The listing builds one solid part. Answer for the finished solid, in the listing's coordinates (mm). Give positions to 0.01 mm unless a question says otherwise; leave off trailing zeros. Order: outer loops, then holes, each group sorted by start corner. A loop starts at its lowest first (then second) coordinate and runs counter-clockwise, first axis right, second up.
```python
from build123d import *

# Parameters (mm, degrees)
SKETCH1_W           = 58
SKETCH1_H           = 61
SKETCH1_R           = 18
BOSS_EXTRUDE1_DEPTH = 8
SKETCH26_R          = 12.25
SKETCH26_R_2        = 3.500000003
SKETCH26_R_3        = 2.7
CUT_EXTRUDE25_DEPTH = 80


with BuildPart() as part:
    # Sketch1 → Boss-Extrude1 (new body)
    with BuildSketch(Plane.XY):
        with Locations((-375.83204095, -9.5)):
            Rectangle(SKETCH1_W, SKETCH1_H)
        with Locations((-375.83204095, -9.5)):
            Circle(SKETCH1_R, mode=Mode.SUBTRACT)
    extrude(amount=BOSS_EXTRUDE1_DEPTH)

    # Sketch26 → Cut-Extrude25 (cut)
    with BuildSketch(Plane(origin=(-392.722155748, 41.581437247, 68), x_dir=(-1, 0, 0), z_dir=(0, 0, 1))):
        with Locations((-16.890114798, 51.081437247)):
            Circle(SKETCH26_R)
        with Locations(Location((-38.640114797, 75.581437247, 0), (0, 0, 180))):
            Circle(SKETCH26_R_2)
        with Locations(Location((4.859885202, 75.581437247, 0), (0, 0, 180))):
            Circle(SKETCH26_R_2)
        with Locations(Location((-38.640114797, 26.581437247, 0), (0, 0, 180))):
            Circle(SKETCH26_R_2)
        with Locations(Location((4.859885202, 26.581437247, 0), (0, 0, 180))):
            Circle(SKETCH26_R_2)
        with Locations((-16.890114798, 16.121848563)):
            Circle(SKETCH26_R_3)
    extrude(amount=-CUT_EXTRUDE25_DEPTH, mode=Mode.SUBTRACT)


solid = part.part
```
1) Find section A-A (y = -9.5). Write down the section's boundary in (x, z).
Geometry says:
outline: (-404.83, 0) - (-393.83, 0) - (-393.83, 8) - (-404.83, 8) - close; (-357.83, 0) - (-346.83, 0) - (-346.83, 8) - (-357.83, 8) - close
2) Find section B-B (y = 15). Write down the section's boundary in (x, z).
Geometry says:
outline: (-404.83, 0) - (-401.08, 0) - (-401.08, 8) - (-404.83, 8) - close; (-394.08, 0) - (-357.58, 0) - (-357.58, 8) - (-394.08, 8) - close; (-350.58, 0) - (-346.83, 0) - (-346.83, 8) - (-350.58, 8) - close
3) Straight lines are drawn through the part: probe 1 along X at (y, z) = (12, 1); probe 2 along Y at (x, z) = (-394.5, 3.5); probe 3 along X at (y, z) = (14.5, 2). For each, find the intervals that lie inside material, in ascending order.
Geometry says:
probe 1: x = -404.83 to -399.38, -395.78 to -355.88, -352.28 to -346.83
probe 2: y = -40 to -35.66, -32.34 to 13.34, 16.66 to 21
probe 3: x = -404.83 to -401.05, -394.12 to -357.55, -350.62 to -346.83
4) Find section D-D (z = 1.75). Write down the section's boundary in (x, y).
Geometry says:
outline: (-404.83, -40) - (-346.83, -40) - (-346.83, 21) - (-404.83, 21) - close; hole circle Ø7 at (-397.58, -34); hole circle Ø7 at (-397.58, 15); hole circle Ø36 at (-375.83, -9.5); hole circle Ø7 at (-354.08, -34); hole circle Ø7 at (-354.08, 15)
5) For a pull along Y with two mould halves and no side action, classify faces 1 (the flat face through (-363, 4, 8)), 2 (the flat face through (-376, 21, 4)), 3 (the cylindrical face through (-393.815, -8.709, 3.944)) as +Y half, -Y half, draft (parallel to the pull), parting line (faces both ways), or undercut.
Geometry says:
face 1: draft
face 2: +Y half
face 3: undercut
6) Find section C-C (x = -370). Write down the section's boundary in (y, z).
Geometry says:
outline: (-40, 0) - (-26.53, 0) - (-26.53, 8) - (-40, 8) - close; (7.53, 0) - (21, 0) - (21, 8) - (7.53, 8) - close
